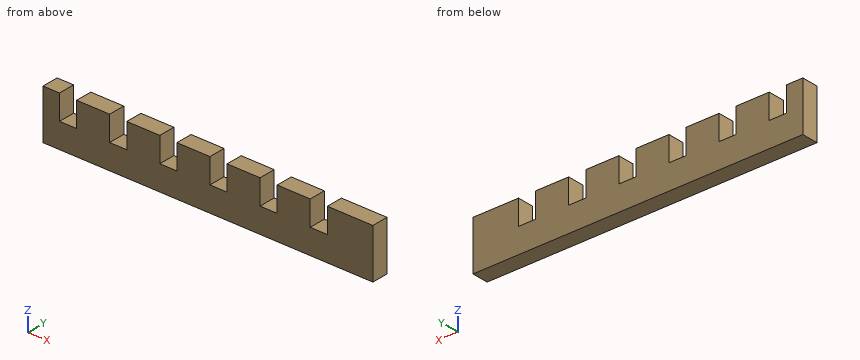
```python
from build123d import *

# Parameters (mm, degrees)
SKETCH1_W           = 100
SKETCH1_H           = 15
BOSS_EXTRUDE1_DEPTH = 5
SKETCH2_W           = 5.2
SKETCH2_H           = 7.5
CUT_EXTRUDE1_DEPTH  = 5


with BuildPart() as part:
    # Sketch1 → Boss-Extrude1 (new body)
    with BuildSketch(Plane(origin=(0, 0, 0), x_dir=(1, 0, 0), z_dir=(0, 1, 0))):
        Rectangle(SKETCH1_W, SKETCH1_H)
    extrude(amount=BOSS_EXTRUDE1_DEPTH)

    # Sketch2 → Cut-Extrude1 (cut)
    with BuildSketch(Plane(origin=(0, 0, 0), x_dir=(1, 0, 0), z_dir=(0, 1, 0))):
        with Locations((-42.4, -3.75)):
            Rectangle(SKETCH2_W, SKETCH2_H)
        with Locations((-27.2, -3.75)):
            Rectangle(SKETCH2_W, SKETCH2_H)
        with Locations((-12, -3.75)):
            Rectangle(SKETCH2_W, SKETCH2_H)
        with Locations((3.2, -3.75)):
            Rectangle(SKETCH2_W, SKETCH2_H)
        with Locations((18.4, -3.75)):
            Rectangle(SKETCH2_W, SKETCH2_H)
        with Locations((33.6, -3.75)):
            Rectangle(SKETCH2_W, SKETCH2_H)
    extrude(amount=CUT_EXTRUDE1_DEPTH, mode=Mode.SUBTRACT)


solid = part.part
```
Geometry: final body of the model. Coordinates: model frame, mm. Round coordinates to 2 decimals unless told otherwise and drop trailing zeros. Order: outer loops, then holes, each group sorted by start corner. A loop starts at its lowest first (then second) coordinate and runs counter-clockwise, first axis right, second up. Notation, with made-up numbers: (-6.5, 44.5) -> (24.5, 44.5) arc R18 cw to (24.5, 57.5) -> close; hole circle Ø11 at (3.25, 13.25). An arc over 180 degrees is marked (long way). Use one line per item in the form item = value. Start each with the question number.
1. Pin query (flat end, axial travel): pin 1 Ø1.5 at (x, y) = (-42, 1.5) entering from +Z. Return the tip coordinate at first contact, or that it passes through.
2. Line query: probe 1 along Z at (x, y) = (33, 2). Output: solid intervals per line, ascending.
3. Cut plane B-B (y = 3.5). Return the cut outline in (x, z), then the cut area to 3 significant figures.
4. Cut plane C-C (x = -12.5). Return the cut outline in (y, z).
5. Cut plane A-A (z = 6.5). Return the cut outline in (x, y).
Solution:
q1.pin_1 = 0
q2.probe_1 = -7.5 to 0
q3.outline = (-50, -7.5) -> (50, -7.5) -> (50, 7.5) -> (36.2, 7.5) -> (36.2, 0) -> (31, 0) -> (31, 7.5) -> (21, 7.5) -> (21, 0) -> (15.8, 0) -> (15.8, 7.5) -> (5.8, 7.5) -> (5.8, 0) -> (0.6, 0) -> (0.6, 7.5) -> (-9.4, 7.5) -> (-9.4, 0) -> (-14.6, 0) -> (-14.6, 7.5) -> (-24.6, 7.5) -> (-24.6, 0) -> (-29.8, 0) -> (-29.8, 7.5) -> (-39.8, 7.5) -> (-39.8, 0) -> (-45, 0) -> (-45, 7.5) -> (-50, 7.5) -> close
q3.area = 1,270 mm^2
q4.outline = (0, -7.5) -> (5, -7.5) -> (5, 0) -> (0, 0) -> close
q5.outline = (-50, 0) -> (-45, 0) -> (-45, 5) -> (-50, 5) -> close; (-39.8, 0) -> (-29.8, 0) -> (-29.8, 5) -> (-39.8, 5) -> close; (-24.6, 0) -> (-14.6, 0) -> (-14.6, 5) -> (-24.6, 5) -> close; (-9.4, 0) -> (0.6, 0) -> (0.6, 5) -> (-9.4, 5) -> close; (5.8, 0) -> (15.8, 0) -> (15.8, 5) -> (5.8, 5) -> close; (21, 0) -> (31, 0) -> (31, 5) -> (21, 5) -> close; (36.2, 0) -> (50, 0) -> (50, 5) -> (36.2, 5) -> close
